Work out the finished part from the listing and answer in its coordinate system (mm). Face numbers are marked on the shaded views. A direction names the side the tool comes from. Round coordinates to 2 decimals unless told otherwise and drop trailing zeros. Loops run counter-clockwise (first coordinate to the right, second up) from the corner with the lowest first, then second, coordinate; pieces in that order, holes last. Notation, with made-up numbers: (-12, 35) - (24, 35) arc R25 ccw to (24, 56) - close; hole circle Ø5 at (-24.75, 4). An arc over 180 degrees is marked (long way). Return JSON: item names as keys, results as strings.
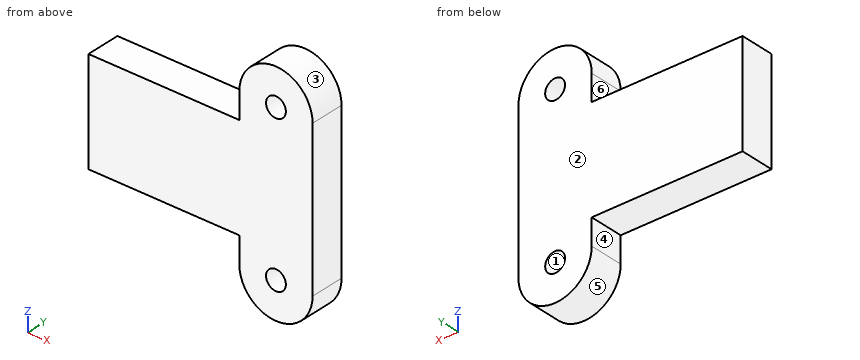
from build123d import *

# Parameters (mm, degrees)
ESBO_O1_R                = 1.15
RESSALTO_EXTRUS_O1_DEPTH = 4


with BuildPart() as part:
    # Esboço1 → Ressalto-extrusão1 (new body)
    with BuildSketch(Plane(origin=(0, 0, 0), x_dir=(1, 0, 0), z_dir=(0, 1, 0))):
        with BuildLine():
            Line((-8.5, 9), (-8.5, 6))
            Line((-8.5, 6), (-26, 6))
            Line((-26, 6), (-26, -6))
            Line((-26, -6), (-8.5, -6))
            Line((-8.5, -6), (-8.5, -9))
            ThreePointArc((-8.5, -9), (-4.25, -13.25), (0, -9))
            Line((0, -9), (0, 9))
            ThreePointArc((0, 9), (-4.25, 13.25), (-8.5, 9))
        make_face()
        with Locations(Location((-4.25, 9, 0), (0, 0, 270))):
            Circle(ESBO_O1_R, mode=Mode.SUBTRACT)
        with Locations(Location((-4.25, -9, 0), (0, 0, 270))):
            Circle(ESBO_O1_R, mode=Mode.SUBTRACT)
    extrude(amount=RESSALTO_EXTRUS_O1_DEPTH)


solid = part.part
1) Section A-A (y = 3.65) is taken. Give the vertices of the cut face in (x, z).
Verdict:
{"outline": "(-26, -6) - (-8.5, -6) - (-8.5, -9) arc R4.25 ccw to (0, -9) - (0, 9) arc R4.25 ccw to (-8.5, 9) - (-8.5, 6) - (-26, 6) - close; hole circle Ø2.3 at (-4.25, -9); hole circle Ø2.3 at (-4.25, 9)"}
2) Determine the mould class of the marked faces 1, 2 and 3 for opening direction X: pulls with the +X half, pulls with the -X half, needs draft (parallel to the pull), parting line crosses it, or undercut.
Verdict:
{"face 1": "undercut", "face 2": "needs draft", "face 3": "parting line crosses it"}
3) Find the intervals of material crossed by L1, parallel to X at y = 2.65, z = 9; L2, parallel to Z at x = -11.25, y = 3.45; L3, parallel to X at y = 0.35, z = 6.5, in increasing order.
Verdict:
{"L1": "x = -8.5 to -5.4, -3.1 to 0", "L2": "z = -6 to 6", "L3": "x = -8.5 to 0"}
4) Section D-D (x = -9) is taken. Give the vertices of the cut face in (y, z).
Verdict:
{"outline": "(0, -6) - (4, -6) - (4, 6) - (0, 6) - close"}
5) Section C-C (z = 6.5) is taken. Give the vertices of the cut face in (x, y), and give its area (3 significant figures).
Verdict:
{"outline": "(-8.5, 0) - (0, 0) - (0, 4) - (-8.5, 4) - close", "area": "34.0 mm2"}
6) Flat-ended cylindrical pins translate along their axes: pin 1 (1 mm diameter, centred on y = 3.5, z = -7.5, fed in from -X); pin 2 (2 mm diameter, centred on x = -20, y = 1, fed in from +Z). Find the tip coordinate at first contact, or state that the pin passes through.
Verdict:
{"pin 1": "stops at x = -8.5", "pin 2": "stops at z = 6"}
7) A tool of negligible diameter and unlimited length cuts with its end or side. For the marked faces 4, 5 and 6, from which of +Z, -Z, +X, -X, +Y, -Y can it reach the whole face along a straight path? Write none if from no direction.
Verdict:
{"face 4": "-Z, -X, +Y, -Y", "face 5": "-Z, +Y, -Y", "face 6": "+Z, -X, +Y, -Y"}
8) Section B-B (x = -4.25) is taken. Give the vertices of the cut face in (y, z).
Verdict:
{"outline": "(0, -13.25) - (4, -13.25) - (4, -10.15) - (0, -10.15) - close; (0, -7.85) - (4, -7.85) - (4, 7.85) - (0, 7.85) - close; (0, 10.15) - (4, 10.15) - (4, 13.25) - (0, 13.25) - close"}
